Could you check a few things on this model? Use its own coordinates, in mm. Give positions to 0.01 mm unless a question says otherwise; leave off trailing zeros. Order: outer loops, then holes, each group sorted by start corner. A loop starts at its lowest first (then second) coordinate and runs counter-clockwise, first axis right, second up.
(1) Imagine slicing it at B-B, the plane x = 0. Write out the boundary of the cut face in (y, z).
(2) Imagine slicing it at C-C, the plane y = 14.25. Write out the boundary of the cut face in (x, z).
(3) Imagine slicing it at A-A, the plane z = 0. Write out the boundary of the cut face in (x, y).
(4) If I drill on probe 1 along X at (y, z) = (18, 0); probe 2 along Z at (x, y) = (0, 6.25); probe 3 along Z at (x, y) = (0, 9), over which ranges is the centre line in solid material (lowest first)?
(5) Imagine slicing it at D-D, the plane z = -18. Write out the boundary of the cut face in (x, y).
(6) Will these pins go through, and if not, where does the flat tip stop? pin 1 (1 mm diameter, centred on x = 0, y = 13.5, fed in from +Z); pin 2 (1 mm diameter, centred on x = -8, z = -14, fed in from -Y); pin 3 (1.5 mm diameter, centred on x = -5.5, y = 5.5, fed in from +Z).
(7) If we mould it in two halves opening along Z, with no side actions, what happens to faces 1 (the cylindrical face through (6.2, 11.66, -1.95)), 2 (the flat face through (-0.2, 11.7, 16.2)), 3 (the flat face through (-0.2, 11.3, -15.8)), 4 (the flat face through (-14, 14, 0))? For each: released by +Z, released by -Z, zero draft, split by the parting line, or undercut.
Autodesk Inventor part; units mm, degrees
ref_plane "YZ Plane" through (0, 0, 0) normal (1, 0, 0) x (0, 1, 0)
ref_plane "XZ Plane" through (0, 0, 0) normal (0, 1, 0) x (-1, 0, 0)
ref_plane "XY Plane" through (0, 0, 0) normal (0, 0, 1) x (1, 0, 0)
sketch "Sketch1" plane through (0, 0, 0) normal (1, 0, 0) x (0, 1, 0)
  line L0 (0, 4.5) -> (0, -4.5)
  line L1 (0, -4.5) -> (23, -27.5)
  line L2 (23, -27.5) -> (23, 27.5)
  line L3 (23, 27.5) -> (0, 4.5)
  point P0 (0, 0)
  point P1 (0, 0)
  point P2 (23, 0)
  dimension "d0" = 45
  dimension "d1" = 55
  dimension "d2" = 23
extrude "Extrusion1" add sketch "Sketch1" along normal mid plane 28
sketch "Sketch2" plane through (-14, 23, 27.5) normal (0, 1, 0) x (1, 0, 0)
  circle A0 centre (14, 27.5) radius 6.5
  dimension "d5" = 13
extrude "Extrusion2" cut sketch "Sketch2" against normal through all
properties part number "buttom_camera_fix"
Answer block:
1. outline: (2, -6.5) - (23, -27.5) - (23, -6.5) - close; (2, 6.5) - (23, 6.5) - (23, 27.5) - close
2. outline: (-14, -18.75) - (14, -18.75) - (14, 18.75) - (-14, 18.75) - close; hole circle Ø13 at (0, 0)
3. outline: (-14, 0) - (-6.5, 0) - (-6.5, 23) - (-14, 23) - close; (6.5, 0) - (14, 0) - (14, 23) - (6.5, 23) - close
4. probe 1: x = -14 to -6.5, 6.5 to 14
4. probe 2: z = -10.75 to -6.5, 6.5 to 10.75
4. probe 3: z = -13.5 to -6.5, 6.5 to 13.5
5. outline: (-14, 13.5) - (14, 13.5) - (14, 23) - (-14, 23) - close
6. pin 1: stops at z = 18.5
6. pin 2: stops at y = 9
6. pin 3: stops at z = 10.75
7. face 1: undercut
7. face 2: released by +Z
7. face 3: released by -Z
7. face 4: zero draft
